```python
from build123d import *

# Parameters (mm, degrees)
SKETCH005_W     = 266
SKETCH005_H     = 55
PAD002_DEPTH    = 4
SKETCH023_W     = 40
SKETCH023_H     = 30
POCKET006_DEPTH = 4.001
POCKET013_DEPTH = 4.001
SKETCH039_R     = 3.3
HOLE004_DEPTH   = 4.001


with BuildPart() as part:
    # Sketch005 (on DatumPlane) → Pad002 (new body)
    with BuildSketch(Plane.XZ.offset(-83)):
        with Locations((0, 19.5)):
            Rectangle(SKETCH005_W, SKETCH005_H)
    extrude(amount=PAD002_DEPTH)

    # Sketch023 (on Face5 of Pad002) → Pocket006 (cut, through all)
    with BuildSketch(Plane(origin=(0, 83, 0), x_dir=(1, 0, 0), z_dir=(0, 1, 0))):
        Polygon((-145, 30), (-100, 30), (-100, 0), (-125, 0), (-125, -15.5), (-155, -15.5), (-155, 4.5), (-145, 4.5), align=None)
        with Locations((-40, 15)):
            Rectangle(SKETCH023_W, SKETCH023_H)
        with Locations((40, 15)):
            Rectangle(SKETCH023_W, SKETCH023_H)
        Polygon((100, 30), (145, 30), (145, 4.5), (155, 4.5), (155, -15.5), (125, -15.5), (125, 0), (100, 0), align=None)
        Polygon((-125, -43), (-100, -43), (-100, -73), (-145, -73), (-145, -47.5), (-155, -47.5), (-155, -27.5), (-125, -27.5), align=None)
        with Locations((-40, -58)):
            Rectangle(SKETCH023_W, SKETCH023_H)
        with Locations((40, -58)):
            Rectangle(SKETCH023_W, SKETCH023_H)
        Polygon((100, -43), (125, -43), (125, -27.5), (155, -27.5), (155, -47.5), (145, -47.5), (145, -73), (100, -73), align=None)
    extrude(amount=-POCKET006_DEPTH, mode=Mode.SUBTRACT)

    # Sketch030 (on Face2 of Pocket006) → Pocket013 (cut, through all)
    with BuildSketch(Plane(origin=(0, 83, 0), x_dir=(1, 0, 0), z_dir=(0, 1, 0))):
        with BuildLine():
            Line((-120, -3), (-66, -3))
            ThreePointArc((-64, -5), (-64.585786, -3.585786), (-66, -3))
            Line((-64, -5), (-64, -36))
            ThreePointArc((-66, -38), (-64.585786, -37.414214), (-64, -36))
            Line((-66, -38), (-120, -38))
            ThreePointArc((-122, -36), (-121.414214, -37.414214), (-120, -38))
            Line((-122, -36), (-122, -5))
            ThreePointArc((-120, -3), (-121.414214, -3.585786), (-122, -5))
        make_face()
    extrude(amount=-POCKET013_DEPTH, mode=Mode.SUBTRACT)

    # Sketch039 (on Face2 of Pocket013) → Hole004 (cut, through all)
    with BuildSketch(Plane(origin=(0, 83, 0), x_dir=(1, 0, 0), z_dir=(0, 1, 0))):
        with Locations((39.5, -27)):
            Circle(SKETCH039_R)
    extrude(amount=-HOLE004_DEPTH, mode=Mode.SUBTRACT)


solid = part.part
```
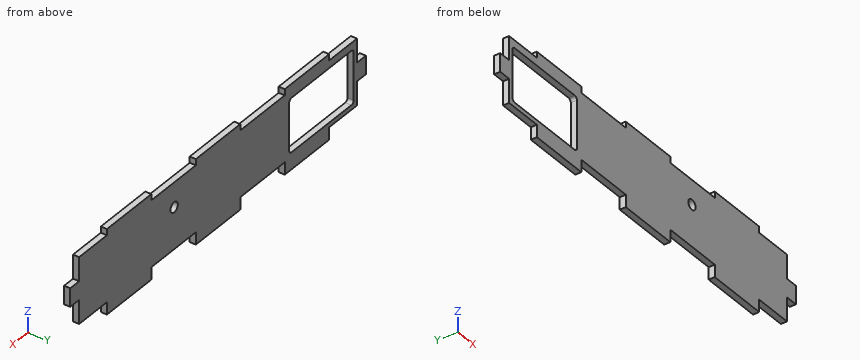
The model under review builds one solid part; all positions refer to its coordinate system, in mm. Round coordinates to 2 decimals unless told otherwise and drop trailing zeros. Write each loop counter-clockwise with the first axis right and the second up, starting at its lowest first coordinate (ties: lowest second). Pieces come first, ordered by that corner, then holes.
(1) Insertion check: pin 1 (1.5 mm diameter, centred on y = 80.5, z = 0.5, fed in from +X); pin 2 (1.2 mm diameter, centred on y = 82, z = -5.5, fed in from +X); pin 3 (2 mm diameter, centred on y = 81.5, z = 45, fed in from -X). Each pin has a flat end and moves straight along its axis. Give the tip position at first contact, or say it passes through.
(2) We need section C-C on y = 80.15. Give the number of separate pieces and of enclosed holes in the cut face, and give its area (3 significant figures).
(3) Wall thickness on L1, parallel to X at y = 80.4, z = 27; L2, parallel to X at y = 82.6, z = 5; L3, parallel to Z at x = -120, y = 82.1: over which ranges is each line inside the solid? List them lowest first.
(4) We need section A-A on z = 19.5. Give the boundary of the cut face in (x, y).
(5) We need section B-B on x = 39.5. Give the boundary of the cut face in (y, z).
(6) We need section D-D on x = -41. Give the boundary of the cut face in (y, z).
Findings below:
1. pin 1: stops at x = 125
1. pin 2: stops at x = 100
1. pin 3: stops at x = -100
2. separate pieces: 1
2. enclosed holes: 2
2. area: 10,300 mm2
3. L1: x = -133 to -122, -64 to 36.2, 42.8 to 133
3. L2: x = -125 to -122, -64 to 125
3. L3: z = 0 to 3, 38 to 43
4. outline: (-133, 79) - (-122, 79) - (-122, 83) - (-133, 83) - close; (-64, 79) - (133, 79) - (133, 83) - (-64, 83) - close
5. outline: (79, 0) - (83, 0) - (83, 23.7) - (79, 23.7) - close; (79, 30.3) - (83, 30.3) - (83, 43) - (79, 43) - close
6. outline: (79, 0) - (83, 0) - (83, 43) - (79, 43) - close
